Input: part model. Units: mm. Frame: model coordinates. A direction names the side the tool comes from. Coordinates: 2 decimals unless noted, no trailing zeros. Order: outer loops, then holes, each group sorted by start corner. A loop starts at its lowest first (then second) coordinate and runs counter-clockwise, first axis right, second up.
from build123d import *

# Parameters (mm, degrees)
BOSS_EXTRUDE3_DEPTH  = 10
SKETCH4_R            = 15
BOSS_EXTRUDE4_DEPTH  = 5
BOSS_EXTRUDE5_START  = 40
BOSS_EXTRUDE5_DEPTH  = 40
SKETCH8_R            = 6.1
BOSS_EXTRUDE10_DEPTH = 10
BOSS_EXTRUDE12_DEPTH = 25.25
BOSS_EXTRUDE13_DEPTH = 18.25
SKETCH13_W           = 49.5
SKETCH13_H           = 5
BOSS_EXTRUDE14_DEPTH = 18.25
SKETCH5_R            = 2.1
SKETCH5_R_2          = 3.25
SKETCH5_R_3          = 4
CUT_EXTRUDE5_DEPTH   = 18.25
SKETCH14_R           = 5.2
BOSS_EXTRUDE15_DEPTH = 10


with BuildPart() as part:
    # Sketch1 → Boss-Extrude3 (new body)
    with BuildSketch(Plane(origin=(0, 0, 0), x_dir=(1, 0, 0), z_dir=(0, 1, 0))):
        with BuildLine():
            Line((0, 37), (100, 37))
            Line((100, 37), (136.997861734, 37))
            Line((136.997861734, 37), (136.997861734, -37))
            Line((136.997861734, -37), (100, -37))
            Line((100, -37), (0, -37))
            ThreePointArc((0, -37), (-37, 0), (0, 37))
        make_face()
    extrude(amount=BOSS_EXTRUDE3_DEPTH)

    # Sketch4 → Boss-Extrude4 (add)
    with BuildSketch(Plane(origin=(0, 10, 0), x_dir=(1, 0, 0), z_dir=(0, 1, 0))):
        with Locations(Location((0, 0, 0), (0, 0, 270))):
            Circle(SKETCH4_R)
    extrude(amount=BOSS_EXTRUDE4_DEPTH)

    # Sketch7 → Boss-Extrude5 (add)
    with BuildSketch(Plane.XZ.offset(BOSS_EXTRUDE5_START)):
        with BuildLine():
            Line((0, -37), (136.997861734, -37))
            Line((136.997861734, -37), (136.997861734, 37))
            Line((136.997861734, 37), (0, 37))
            ThreePointArc((0, 37), (-37, 0), (0, -37))
        make_face()
        with BuildLine():
            ThreePointArc((0, 33), (-33, 0), (0, -33))
            Line((0, -33), (133, -33))
            Line((133, -33), (133, 33))
            Line((133, 33), (0, 33))
        make_face(mode=Mode.SUBTRACT)
    extrude(amount=-BOSS_EXTRUDE5_DEPTH)

    # Sketch8 → Boss-Extrude10 (add)
    # profile 1 of 2: a face of its own
    with BuildSketch(Plane.XZ):
        Polygon((83.5, 33), (83.5, 24), (83.5, 14.75), (100, 14.75), (116.5, 14.75), (116.5, 33), align=None)
        with Locations(Location((100, 24, 0), (0, 0, 270))):
            Circle(SKETCH8_R, mode=Mode.SUBTRACT)
    # profile 2 of 2: a face of its own
    with BuildSketch(Plane.XZ):
        Polygon((83.5, -14.75), (83.5, -30.5), (83.5, -33), (116.5, -33), (116.5, -30.5), (116.5, -14.75), (100, -14.75), align=None)
        with Locations(Location((100, -24, 0), (0, 0, 270))):
            Circle(SKETCH8_R, mode=Mode.SUBTRACT)
    extrude(amount=BOSS_EXTRUDE10_DEPTH)

    # Sketch12 → Boss-Extrude12 (add)
    with BuildSketch(Plane.XZ.offset(10)):
        Polygon((90, 14.75), (90, 24), (90, 33), (83.5, 33), (83.5, 14.75), align=None)
        Polygon((116.5, 33), (110, 33), (110, 24), (110, 14.75), (116.5, 14.75), align=None)
        Polygon((110, -14.75), (110, -24), (110, -33), (116.5, -33), (116.5, -14.75), align=None)
        Polygon((90, -24), (90, -14.75), (83.5, -14.75), (83.5, -33), (90, -33), align=None)
    extrude(amount=BOSS_EXTRUDE12_DEPTH)

    # Sketch9 → Boss-Extrude13 (add)
    with BuildSketch(Plane(origin=(0, 0, 33), x_dir=(-1, 0, 0), z_dir=(0, 0, -1))):
        Polygon((-133, -35), (-133, -40), (-83.5, -40), (-83.5, -35.25), (-90, -35.25), (-90, -35), (-110, -35), (-110, -35.25), (-116.5, -35.25), (-116.5, -35), align=None)
    extrude(amount=BOSS_EXTRUDE13_DEPTH)

    # Sketch13 → Boss-Extrude14 (add)
    with BuildSketch(Plane.XY.offset(-33)):
        with Locations((108.25, -37.5)):
            Rectangle(SKETCH13_W, SKETCH13_H)
    extrude(amount=BOSS_EXTRUDE14_DEPTH)

    # Sketch5 → Cut-Extrude5 (cut)
    with BuildSketch(Plane.XZ):
        with Locations(Location((-11, 0, 0), (0, 0, 270))):
            Circle(SKETCH5_R)
        with Locations(Location((0, 0, 0), (0, 0, 270))):
            Circle(SKETCH5_R_2)
        with Locations(Location((0, 11, 0), (0, 0, 270))):
            Circle(SKETCH5_R)
        with Locations(Location((11, 0, 0), (0, 0, 270))):
            Circle(SKETCH5_R)
        with Locations(Location((0, -11, 0), (0, 0, 270))):
            Circle(SKETCH5_R)
        with Locations(Location((100, 0, 0), (0, 0, 270))):
            Circle(SKETCH5_R_3)
    extrude(amount=-CUT_EXTRUDE5_DEPTH, mode=Mode.SUBTRACT)

    # Sketch14 → Boss-Extrude15 (add)
    with BuildSketch(Plane.XZ):
        with Locations(Location((100, 24, 0), (0, 0, 90))):
            Circle(SKETCH14_R)
        with Locations(Location((100, -24, 0), (0, 0, 90))):
            Circle(SKETCH14_R)
    extrude(amount=BOSS_EXTRUDE15_DEPTH)


solid = part.part
Item 1: Cut plane D-D on z = 11. Return loops of the section in (x, y), then the cut area to 3 significant figures.
Response values:
outline: (-35.33, -40) - (-31.11, -40) - (-31.11, 0) - (-2.1, 0) - (-2.1, 15) - (-10.2, 15) - (-10.2, 10) - (-35.33, 10) - close; (2.1, 0) - (133, 0) - (133, -40) - (137, -40) - (137, 10) - (10.2, 10) - (10.2, 15) - (2.1, 15) - close
area: 2,090 mm2
Item 2: Cut plane B-B on z = 0. Return loops of the section in (x, y), then the cut area to 3 significant figures.
Response values:
outline: (-37, -40) - (-33, -40) - (-33, 0) - (-13.1, 0) - (-13.1, 15) - (-15, 15) - (-15, 10) - (-37, 10) - close; (-8.9, 0) - (-3.25, 0) - (-3.25, 15) - (-8.9, 15) - close; (3.25, 0) - (8.9, 0) - (8.9, 15) - (3.25, 15) - close; (13.1, 0) - (96, 0) - (96, 10) - (15, 10) - (15, 15) - (13.1, 15) - close; (104, 0) - (133, 0) - (133, -40) - (137, -40) - (137, 10) - (104, 10) - close
area: 1,910 mm2
Item 3: Access query for faces 4 (the face through (41, -20, -33)), 5 (the face through (100, -23, 33)), 6 (the face through (96.451, 4.93, -1.846)). Directions: +Z, -Z, +X, -X, +Y, -Y. A direction counts if a zero-diameter tool reaches every point of the face in a straight line with its end or side. Return the directions, or none.
Response values:
face 4: -Y
face 5: none
face 6: +Y, -Y
Item 4: Cut plane A-A on y = -4. Return loops of the section in (x, z), then the cut area to 3 significant figures.
Response values:
outline: (0, -37) - (137, -37) - (137, 37) - (0, 37) arc R37 ccw to start; circle Ø10.4 at (100, -24); circle Ø10.4 at (100, 24); hole (0, -33) - (83.5, -33) - (83.5, -14.75) - (116.5, -14.75) - (116.5, -33) - (133, -33) - (133, 33) - (116.5, 33) - (116.5, 14.75) - (83.5, 14.75) - (83.5, 33) - (0, 33) arc R33 ccw to start; hole circle Ø12.2 at (100, -24); hole circle Ø12.2 at (100, 24)
area: 2,940 mm2
Item 5: Draft query along Y for faces 1 (the face through (133, -20, 0)), 2 (the face through (114, -20, 14.75)), 3 (the face through (51, 10, -1)). Return one class per face: pulls with the +Y half, pulls with the -Y half, needs draft (parallel to the pull), parting line crosses it, or undercut.
Response values:
face 1: undercut
face 2: needs draft
face 3: pulls with the +Y half
Item 6: Pin query (flat end, axial travel): pin 1 Ø2 at (x, z) = (40.5, -8.5) entering from +Y; pin 2 Ø10 at (x, z) = (6.5, -3.5) entering from -Y; pin 3 Ø7 at (x, z) = (100, 0) entering from -Y; pin 4 Ø1 at (x, y) = (-17, -32.5) entering from -Z. Return the tip coordinate at first contact, or that it passes through.
Response values:
pin 1: stops at y = 10
pin 2: stops at y = 0
pin 3: passes through
pin 4: stops at z = -33.12
Item 7: Cut plane C-C on y = -31.5. Return loops of the section in (x, z), then the cut area to 3 significant figures.
Response values:
outline: (0, -37) - (137, -37) - (137, 37) - (0, 37) arc R37 ccw to start; hole (0, -33) - (83.5, -33) - (83.5, -14.75) - (90, -14.75) - (90, -33) - (110, -33) - (110, -14.75) - (116.5, -14.75) - (116.5, -33) - (133, -33) - (133, 33) - (116.5, 33) - (116.5, 14.75) - (110, 14.75) - (110, 33) - (90, 33) - (90, 14.75) - (83.5, 14.75) - (83.5, 33) - (0, 33) arc R33 ccw to start
area: 2,270 mm2
Item 8: Ray query, probe 1 along X at (y, z) = (11.5, 0); probe 2 along X at (y, z) = (5.75, 0); probe 3 along Z at (x, y) = (74.5, -3). Return the intervals inside material, ascending.
Response values:
probe 1: x = -15 to -13.1, -8.9 to -3.25, 3.25 to 8.9, 13.1 to 15
probe 2: x = -37 to -13.1, -8.9 to -3.25, 3.25 to 8.9, 13.1 to 96, 104 to 137
probe 3: z = -37 to -33, 33 to 37
